Input: dimensioned drawing with shaded views. Units: mm. Origin: part minimum x, y, z. A direction names the side the tool comes from. Give positions to 0.01 mm unless a question says otherwise; leave off trailing zeros. Loops run counter-clockwise (first coordinate to the right, second up) from the corner with the lowest first, then second, coordinate; pieces in that order, holes last.
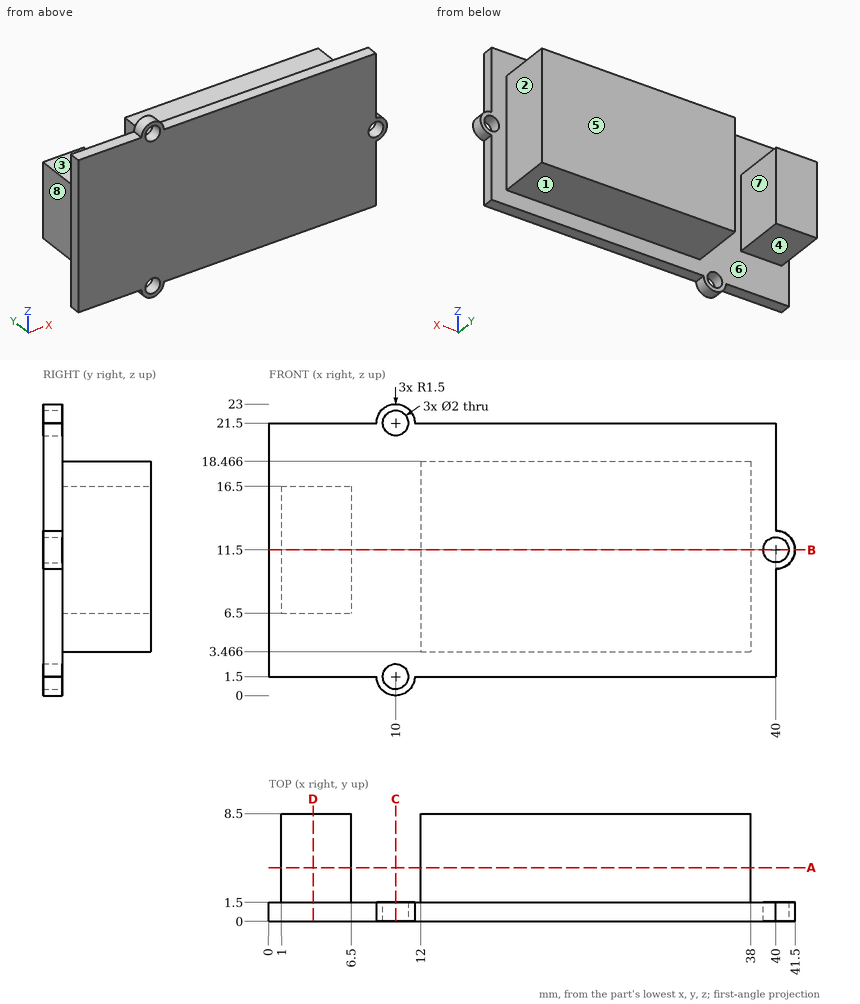
Item 1: Set-up query: the marked faces 1, 2, 3 and 4. Return all of +Z, -Z, +X, -X, +Y, -Y with unobstructed straight access to the full face (end or side cutting, diameter ignored); none if empty.
Values follow:
face 1: -Z, +X, -X, +Y
face 2: +Z, -Z, +X, +Y
face 3: +Z, -X, +Y
face 4: -Z, -X, +Y
Item 2: Section query D-D on x = 3.5. Return loops of the section in (y, z).
Values follow:
outline: (0, 1.5) - (1.5, 1.5) - (1.5, 6.5) - (8.5, 6.5) - (8.5, 16.5) - (1.5, 16.5) - (1.5, 21.5) - (0, 21.5) - close
Item 3: Ray query, probe 1 along Z at (x, y) = (10, 0.9); probe 2 along X at (y, z) = (3.75, 8.25); probe 3 along X at (y, z) = (0.8, 11.5). Return the intervals inside material, ascending.
Values follow:
probe 1: z = 0 to 0.5, 2.5 to 20.5, 22.5 to 23
probe 2: x = 1 to 6.5, 12 to 38
probe 3: x = 0 to 39, 41 to 41.5
Item 4: Section query C-C on x = 10. Return loops of the section in (y, z), plus the area to 3 significant figures.
Values follow:
outline: (0, 0) - (1.5, 0) - (1.5, 0.5) - (0, 0.5) - close; (0, 2.5) - (1.5, 2.5) - (1.5, 20.5) - (0, 20.5) - close; (0, 22.5) - (1.5, 22.5) - (1.5, 23) - (0, 23) - close
area: 28.5 mm2
Item 5: Section query A-A on y = 4.25. Return loops of the section in (x, z).
Values follow:
outline: (1, 6.5) - (6.5, 6.5) - (6.5, 16.5) - (1, 16.5) - close; (12, 3.47) - (38, 3.47) - (38, 18.47) - (12, 18.47) - close
Item 6: Section query B-B on z = 11.5. Return loops of the section in (x, y).
Values follow:
outline: (0, 0) - (39, 0) - (39, 1.5) - (38, 1.5) - (38, 8.5) - (12, 8.5) - (12, 1.5) - (6.5, 1.5) - (6.5, 8.5) - (1, 8.5) - (1, 1.5) - (0, 1.5) - close; (41, 0) - (41.5, 0) - (41.5, 1.5) - (41, 1.5) - close
Item 7: Draft query along X for the marked faces 5, 6, 7 and 8. Return one class per face: +X half, -X half, draft (parallel to the pull), parting line (faces both ways), or undercut.
Values follow:
face 5: draft
face 6: undercut
face 7: undercut
face 8: -X half
Item 8: Pin query (flat end, axial travel): pin 1 (2 mm diameter, centred on y = 5.5, z = 11.5, fed in from +X); pin 2 (1.6 mm diameter, centred on y = 0.5, z = 16, fed in from +X); pin 3 (2 mm diameter, centred on y = 3, z = 13, fed in from -X). Return the tip coordinate at first contact, or that it passes through.
Values follow:
pin 1: stops at x = 38
pin 2: stops at x = 40
pin 3: stops at x = 1
